Work out the finished part from the listing and answer in its coordinate system (mm). Round coordinates to 2 decimals unless told otherwise and drop trailing zeros. Write each loop counter-clockwise with the first axis right and the second up, starting at its lowest first coordinate (ties: lowest second). Pieces come first, ordered by that corner, then holes.
1. Straight lines are drawn through the part: probe 1 along Z at (x, y) = (40, 0.7); probe 2 along X at (y, z) = (1.1, -35); probe 3 along Z at (x, y) = (63.9, 0.5). For each, find the intervals that lie inside material, in ascending order.
2. A flat-ended cylindrical pin translates along its axis: pin 1 Ø4 at (x, z) = (40, 35) entering from -Y. Find the tip coordinate at first contact, or state that the pin passes through.
3. Determine the mould class of faces 1 (the face through (85.89, 1.01, 42.15)), 2 (the face through (-1, 0, -1)), 3 (the face through (-0.54, 0.99, -32.56)), 4 (the face through (-61.59, 0.99, 11.54)) for opening direction X: pulls with the +X half, pulls with the -X half, needs draft (parallel to the pull), parting line crosses it, or undercut.
4. Find section B-B (x = 0). Write down the section's boundary in (y, z).
5. Find section A-A (y = 1.55). Count the separate pieces of the cut face and the enclosed holes in it, and give its area (3 significant figures).
```python
from build123d import *

# Parameters (mm, degrees)
SKETCH1_W           = 177.8
SKETCH1_H           = 90
SKETCH1_R           = 2.5
BOSS_EXTRUDE1_DEPTH = 2
FILLET1_R           = 10
SKETCH2_R           = 2.5
SKETCH2_R_2         = 1.5
CUT_EXTRUDE1_DEPTH  = 2


with BuildPart() as part:
    # Sketch1 → Boss-Extrude1 (new body)
    with BuildSketch(Plane(origin=(0, 0, 0), x_dir=(1, 0, 0), z_dir=(0, 1, 0))):
        Rectangle(SKETCH1_W, SKETCH1_H)
        with Locations((0, 35)):
            Circle(SKETCH1_R, mode=Mode.SUBTRACT)
        with Locations((0, -35)):
            Circle(SKETCH1_R, mode=Mode.SUBTRACT)
        with Locations((40, 35)):
            Circle(SKETCH1_R, mode=Mode.SUBTRACT)
        with Locations((40, -35)):
            Circle(SKETCH1_R, mode=Mode.SUBTRACT)
        with Locations((-40, 35)):
            Circle(SKETCH1_R, mode=Mode.SUBTRACT)
        with Locations((-40, -35)):
            Circle(SKETCH1_R, mode=Mode.SUBTRACT)
    extrude(amount=BOSS_EXTRUDE1_DEPTH)

    # Fillet1
    fillet1_edges = [part.edges().sort_by_distance(p)[0] for p in [
        (-88.9, 1, 45),
        (-88.9, 1, -45),
        (88.9, 1, -45),
        (88.9, 1, 45),
    ]]
    fillet(fillet1_edges, radius=FILLET1_R)

    # Sketch2 → Cut-Extrude1 (cut)
    with BuildSketch(Plane.XZ):
        with Locations((-63.9, 12.5)):
            Circle(SKETCH2_R)
        with Locations((-63.9, -12.5)):
            Circle(SKETCH2_R)
        with Locations((63.9, 12.5)):
            Circle(SKETCH2_R_2)
        with Locations((63.9, -12.5)):
            Circle(SKETCH2_R_2)
    extrude(amount=-CUT_EXTRUDE1_DEPTH, mode=Mode.SUBTRACT)


solid = part.part
```
Worked answers:
1. probe 1: z = -45 to -37.5, -32.5 to 32.5, 37.5 to 45
1. probe 2: x = -88.9 to -42.5, -37.5 to -2.5, 2.5 to 37.5, 42.5 to 88.9
1. probe 3: z = -45 to -14, -11 to 11, 14 to 45
2. pin 1: passes through
3. face 1: pulls with the +X half
3. face 2: needs draft
3. face 3: undercut
3. face 4: undercut
4. outline: (0, -45) - (2, -45) - (2, -37.5) - (0, -37.5) - close; (0, -32.5) - (2, -32.5) - (2, 32.5) - (0, 32.5) - close; (0, 37.5) - (2, 37.5) - (2, 45) - (0, 45) - close
5. separate pieces: 1
5. enclosed holes: 10
5. area: 15,700 mm2
